The figure shows three views and two pictorial views of one solid part (mm, origin at its lowest corner). Answer the questions. A direction names the side the tool comes from. Coordinates: 2 decimals unless noted, no trailing zeros. Answer in a Markdown table with one row per item.
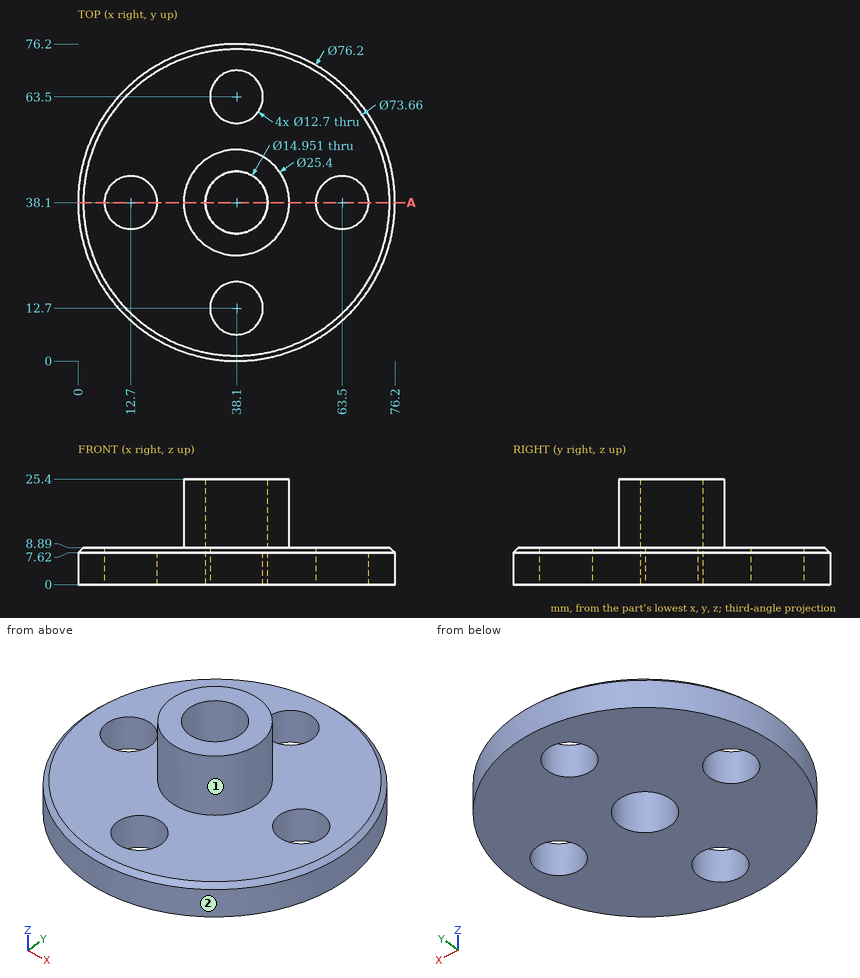
Item 1: Find the intervals of material crossed by probe 1 along Y at (x, z) = (41.5, 4.5); probe 2 along Y at (x, z) = (36, 3.5) (1 decimal); probe 3 along Z at (x, y) = (31.5, 71), in increasing order.
Findings below:
| item | result |
|---|---|
| probe 1 | y = 0.15 to 7.34, 18.06 to 31.44, 44.76 to 58.14, 68.86 to 76.05 |
| probe 2 | y = 0.1 to 6.7, 18.7 to 30.9, 45.3 to 57.5, 69.5 to 76.1 |
| probe 3 | z = 0 to 8.89 |
Item 2: Flat-ended cylindrical pins translate along their axes: pin 1 Ø3 at (x, z) = (43.5, 9.5) entering from -Y (1 decimal); pin 2 Ø2 at (x, y) = (23.5, 38.5) entering from +Z; pin 3 Ø3 at (y, z) = (33, 3) entering from +X; pin 4 Ø10 at (x, y) = (63.5, 38.1) entering from -Z. Find the tip coordinate at first contact, or state that the pin passes through.
Findings below:
| item | result |
|---|---|
| pin 1 | stops at y = 0.8 |
| pin 2 | stops at z = 8.89 |
| pin 3 | stops at x = 76.03 |
| pin 4 | passes through |
Item 3: A tool of negligible diameter and unlimited length cuts with its end or side. For the marked faces 1 and 2, from which of +Z, -Z, +X, -X, +Y, -Y can it reach the whole face along a straight path? Write none if from no direction.
Findings below:
| item | result |
|---|---|
| face 1 | +Z |
| face 2 | +Z, -Z |
Item 4: A cutting plane is placed at A-A, the plane y = 38.1. Count the separate pieces of the cut face and the enclosed holes in it.
Findings below:
| item | result |
|---|---|
| separate pieces | 4 |
| enclosed holes | 0 |
